Part model, mm, in its own coordinate system. Face numbers are marked on the shaded views. A direction names the side the tool comes from. Round coordinates to 2 decimals unless told otherwise and drop trailing zeros. Write each loop counter-clockwise with the first axis right and the second up, starting at its lowest first coordinate (ties: lowest second). Pieces come first, ordered by that corner, then holes. Notation, with made-up numbers: M 45.5,-23 L 92.5,-23 A16 ccw 92.5,3 Z; hole C 38.5,74.25 d4. An arc over 180 degrees is marked long. Use a Markdown table: item, result. Add a question column.
1) Slice it at D-D on z = 2. Write the cut outline in (x, y).
2) Two-plate mould, pull along Z, no slides. Class the marked faces 4, 5 and 6: released by +Z, released by -Z, zero draft, split by the parting line, or undercut.
3) Drop flat-ended pins along their axis: P1, Ø3, axis at x = 10, y = 7, coming from the +Z side; P2, Ø10, axis at y = 3.5, z = -15.5, coming from the -X side; P3, Ø5.5, axis at x = -1, z = 14.5, coming from the -Y side. Give the stop position or say it passes through.
4) Slice it at A-A on x = 0. Write the cut outline in (y, z).
5) Which spindle directions (+Z, -Z, +X, -X, +Y, -Y) get a long thin tool onto all of the face, cutting with end or side? Do the marked faces 1, 2 and 3. Say none if no direction does.
6) Wall check: probe 1 along Y at (x, z) = (-3.75, 11); probe 2 along Z at (x, y) = (2, -1.5); probe 3 along Y at (x, z) = (5, 13). Give the ranges that are in metal, low to high.
7) Slice it at B-B on y = 0. Write the cut outline in (x, z) (3 decimals).
8) Slice it at C-C on y = -6.75. Write the cut outline in (x, z), plus the area to 3 significant figures.
```python
from build123d import *

# Parameters (mm, degrees)
F0_R     = 7.747
F1_DEPTH = 20.32
F0_R_2   = 13.97
F2_DEPTH = 25.4
F3_R     = 13.97
F5_DEPTH = 11.43
F6_R     = 3.175
F7_DEPTH = 6.35


with BuildPart() as f1:
    # F0 (on Top) → F1 (new body)
    with BuildSketch(Plane.XY):
        Circle(F0_R)
    extrude(amount=F1_DEPTH)

    # F0 (on Top) → F2 (join)
    with BuildSketch(Plane.XY):
        Circle(F0_R_2)
        Circle(F0_R, mode=Mode.SUBTRACT)
        Circle(F0_R)
    extrude(amount=-F2_DEPTH)

    # F3
    f3_edges = [f1.edges().sort_by_distance(p)[0] for p in [
        (-13.97, 0, -25.4),
    ]]
    fillet(f3_edges, radius=F3_R)

    # F4 (on face) → F5 (cut)
    with BuildSketch(Plane.XY.offset(20.32)):
        with BuildLine():
            Line((10.1125147194, 5.08), (5.8488981014, 5.08))
            ThreePointArc((5.8488981014, 5.08), (7.2569767325, 2.7115120698), (7.747, 0))
            ThreePointArc((7.747, 0), (7.2569767325, -2.7115120698), (5.8488981014, -5.08))
            Line((5.8488981014, -5.08), (10.1125147194, -5.08))
            Line((10.1125147194, -5.08), (10.1125147194, 5.08))
        make_face()
        with BuildLine():
            Line((5.8488981014, 5.08), (-5.8488981014, 5.08))
            ThreePointArc((-5.8488981014, 5.08), (-7.747, 0), (-5.8488981014, -5.08))
            Line((-5.8488981014, -5.08), (5.8488981014, -5.08))
            ThreePointArc((5.8488981014, -5.08), (7.2569767325, -2.7115120698), (7.747, 0))
            ThreePointArc((7.747, 0), (7.2569767325, 2.7115120698), (5.8488981014, 5.08))
        make_face()
        with BuildLine():
            Line((-5.8488981014, 5.08), (-9.6324700862, 5.08))
            Line((-9.6324700862, 5.08), (-9.6324700862, -5.08))
            Line((-9.6324700862, -5.08), (-5.8488981014, -5.08))
            ThreePointArc((-5.8488981014, -5.08), (-7.747, 0), (-5.8488981014, 5.08))
        make_face()
    extrude(amount=-F5_DEPTH, mode=Mode.SUBTRACT)

    # F6 (on Front) → F7 (join, symmetric)
    with BuildSketch(Plane.XZ):
        with Locations((0, 15.116378665)):
            Circle(F6_R)
    extrude(amount=F7_DEPTH, both=True)


solid = f1.part
```
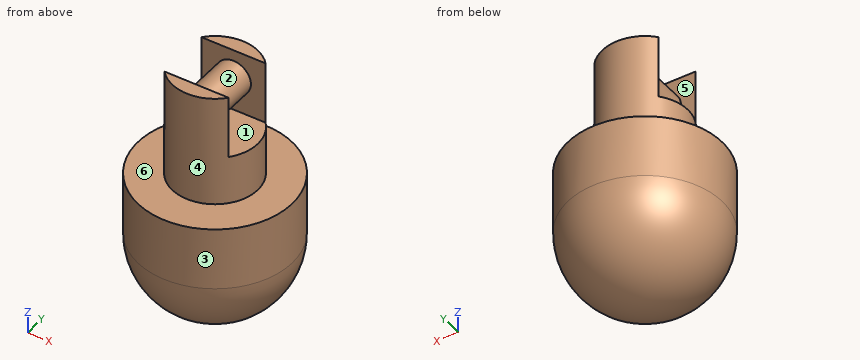
Entries:
| question | item | result |
|---|---|---|
| 1 | outline | C 0,0 d15.49 |
| 2 | face 4 | zero draft |
| 2 | face 5 | undercut |
| 2 | face 6 | released by +Z |
| 3 | P1 | stops at z = 0 |
| 3 | P2 | stops at x = -13.97 |
| 3 | P3 | stops at y = -7.75 |
| 4 | outline | M -13.97,-11.43 A13.97 ccw 13.97,-11.43 L 13.97,0 L 7.75,0 L 7.75,20.32 L 5.08,20.32 L 5.08,18.29 L -5.08,18.29 L -5.08,20.32 L -7.75,20.32 L -7.75,0 L -13.97,0 Z; hole M -5.08,8.89 L 5.08,8.89 L 5.08,11.94 L -5.08,11.94 Z |
| 5 | face 1 | +X, -X |
| 5 | face 2 | none |
| 5 | face 3 | +Z, -Z |
| 6 | probe 1 | y = -6.78 to -5.08, 5.08 to 6.78 |
| 6 | probe 2 | z = -25.17 to 8.89, 12.65 to 17.58 |
| 6 | probe 3 | y = -5.92 to -5.08, 5.08 to 5.92 |
| 7 | outline | M -13.97,-11.43 A13.97 ccw 13.97,-11.43 L 13.97,0 L 7.747,0 L 7.747,8.89 L -7.747,8.89 L -7.747,0 L -13.97,0 Z; C 0,15.116 d6.35 |
| 8 | outline | M -12.23,-11.43 A12.23 ccw 12.23,-11.43 L 12.23,0 L 3.8,0 L 3.8,20.32 L -3.8,20.32 L -3.8,0 L -12.23,0 Z |
| 8 | area | 669 mm^2 |
